Autodesk Inventor part; units mm, degrees
ref_plane "YZ Plane" through (0, 0, 0) normal (1, 0, 0) x (0, 1, 0)
ref_plane "XZ Plane" through (0, 0, 0) normal (0, 1, 0) x (-1, 0, 0)
ref_plane "XY Plane" through (0, 0, 0) normal (0, 0, 1) x (1, 0, 0)
sketch "Sketch1" plane through (0, 0, 0) normal (0, 0, 1) x (1, 0, 0)
  line L0 (-7.5, 16) -> (7.5, 16)
  line L1 (7.5, 16) -> (7.5, -16)
  line L2 (7.5, -16) -> (-7.5, -16)
  line L3 (-7.5, -16) -> (-7.5, 16)
  line L4 (-7.5, 16) -> (7.5, -16) construction
  line L5 (7.5, 16) -> (-7.5, -16) construction
  point P0 (0, 0)
  dimension "d0" = 32
  dimension "d2" = 15
extrude "Extrusion1" add sketch "Sketch1" along normal mid plane 3
sketch "Sketch2" plane through (0, 0, 1.5) normal (0, 0, 1) x (1, 0, 0)
  line L0 (7.5, 16) -> (-7.5, 16)
  line L1 (-7.5, -16) -> (7.5, -16)
  line L2 (0, 16) -> (0, -16) construction
  point P0 (0, 0)
  point P1 (0, 13.5)
  point P2 (0, 3.5)
  point P3 (-5, 8.5)
  point P4 (5, 8.5)
  dimension "d5" = 10
  dimension "d7" = 10
  dimension "d8" = 5
  dimension "d9" = 2.5
  dimension "d10" = 5
hole "Hole1" at (0, 13.5, 1.5) at (0, 3.5, 1.5) at (-5, 8.5, 1.5) at (5, 8.5, 1.5) direction (0, 0, -1) diameter 3 end through all
sketch "Sketch3" plane through (0, 0, 1.5) normal (0, 0, 1) x (1, 0, 0)
  line L0 (-7.5, -16) -> (7.5, -16)
  line L1 (7.5, -16) -> (7.5, 16)
  line L2 (0, -23.093) -> (0, 0) construction
  line L3 (-2.75, -4.73) -> (2.75, -4.73)
  line L4 (2.75, -4.73) -> (2.75, -10.23)
  line L5 (2.75, -10.23) -> (-2.75, -10.23)
  line L6 (-2.75, -10.23) -> (-2.75, -4.73)
  line L7 (-2.75, -4.73) -> (2.75, -10.23) construction
  line L8 (2.75, -4.73) -> (-2.75, -10.23) construction
  arc A0 (-2.75, -10.23) -> (2.75, -10.23) centre (0, -10.23) ccw
  arc A1 (2.75, -4.73) -> (-2.75, -4.73) centre (0, -4.73) ccw
  point P0 (0, -7.48)
  dimension "d18" = 5.5
  dimension "d20" = 5.5
  dimension "d21" = 3.02
extrude "Extrusion2" cut sketch "Sketch3" against normal through all
properties part number "Micro Limit Switch Plate" material "Aluminum 6061"
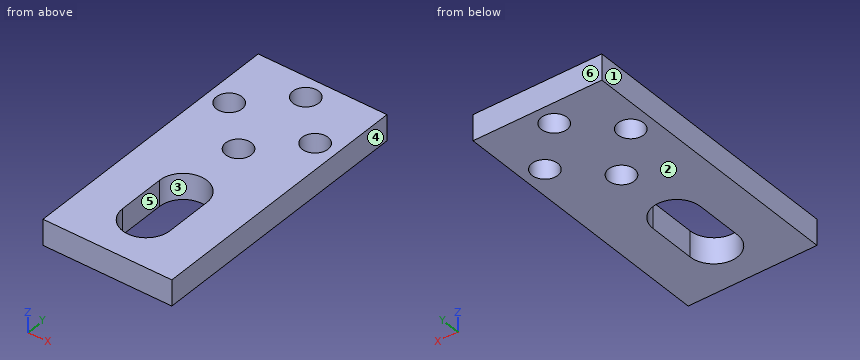
Here's how the part is built. I have some questions about the finished solid (model axes, mm). Face numbers are marked on the shaded views. A direction names the side the tool comes from. Coordinates: 2 decimals unless noted, no trailing zeros. Write each loop counter-clockwise with the first axis right and the second up, starting at its lowest first coordinate (ties: lowest second). Pieces come first, ordered by that corner, then holes. Notation, with made-up numbers: (-3.5, 81) - (42.5, 81) arc R36 ccw to (42.5, 117) - close; hole circle Ø3 at (-17.5, -38). An arc over 180 degrees is marked (long way). One line per item, written item: value.
1) On a 3-axis mill with a long thin cutter (end or side, diameter ignored), from which of +Z, -Z, +X, -X, +Y, -Y can I reach the whole of each face in a straight line? I mean the marked faces 5 and 6. Say none if no direction works.
Model answer:
face 5: +Z, -Z
face 6: +Z, -Z, +X, -X, +Y
2) Suppose I cut it at C-C on z = -0.4. Write out the boundary of the cut face in (x, y), and give its area (3 significant figures).
Model answer:
outline: (-7.5, -16) - (7.5, -16) - (7.5, 16) - (-7.5, 16) - close; hole circle Ø3 at (-5, 8.5); hole (-2.75, -10.23) arc R2.75 ccw to (2.75, -10.23) - (2.75, -4.73) arc R2.75 ccw to (-2.75, -4.73) - close; hole circle Ø3 at (0, 3.5); hole circle Ø3 at (0, 13.5); hole circle Ø3 at (5, 8.5)
area: 398 mm²
3) Suppose I cut it at A-A on x = 5. Write out the boundary of the cut face in (y, z).
Model answer:
outline: (-16, -1.5) - (7, -1.5) - (7, 1.5) - (-16, 1.5) - close; (10, -1.5) - (16, -1.5) - (16, 1.5) - (10, 1.5) - close
4) Suppose I cut it at D-D on y = -7. Write out the boundary of the cut face in (x, z), and give its area (3 significant figures).
Model answer:
outline: (-7.5, -1.5) - (-2.75, -1.5) - (-2.75, 1.5) - (-7.5, 1.5) - close; (2.75, -1.5) - (7.5, -1.5) - (7.5, 1.5) - (2.75, 1.5) - close
area: 28.5 mm²
5) Suppose I cut it at B-B on y = 8.5. Write out the boundary of the cut face in (x, z), and give its area (3 significant figures).
Model answer:
outline: (-7.5, -1.5) - (-6.5, -1.5) - (-6.5, 1.5) - (-7.5, 1.5) - close; (-3.5, -1.5) - (3.5, -1.5) - (3.5, 1.5) - (-3.5, 1.5) - close; (6.5, -1.5) - (7.5, -1.5) - (7.5, 1.5) - (6.5, 1.5) - close
area: 27.0 mm²
6) We'd pull the mould along X, two halves only. Please class the marked faces 1, 2, 3 and 4: pulls with the +X half, pulls with the -X half, needs draft (parallel to the pull), parting line crosses it, or undercut.
Model answer:
face 1: pulls with the -X half
face 2: needs draft
face 3: undercut
face 4: pulls with the +X half
7) I need wall thicknesses on line 1 along Y through (x, z) = (0, 0.5); line 2 along X through (y, z) = (8.5, 0); line 3 along Y through (x, z) = (-5, 0.4). Which ranges of each line are inside material? Lowest first, please.
Model answer:
line 1: y = -16 to -12.98, -1.98 to 2, 5 to 12, 15 to 16
line 2: x = -7.5 to -6.5, -3.5 to 3.5, 6.5 to 7.5
line 3: y = -16 to 7, 10 to 16
